Part print with two shaded views. Sizes in mm from the minimum x, y, z corner. Round coordinates to 2 decimals unless told otherwise and drop trailing zeros. Order: outer loops, then holes, each group sorted by start corner. A loop starts at its lowest first (then second) coordinate and runs counter-clockwise, first axis right, second up. Notation, with made-up numbers: (63, 26.25) - (85, 26.25) arc R28 ccw to (85, 62.25) - close; hole circle Ø4 at (85, 48.25). An arc over 180 degrees is marked (long way). Write item = value, one per line.
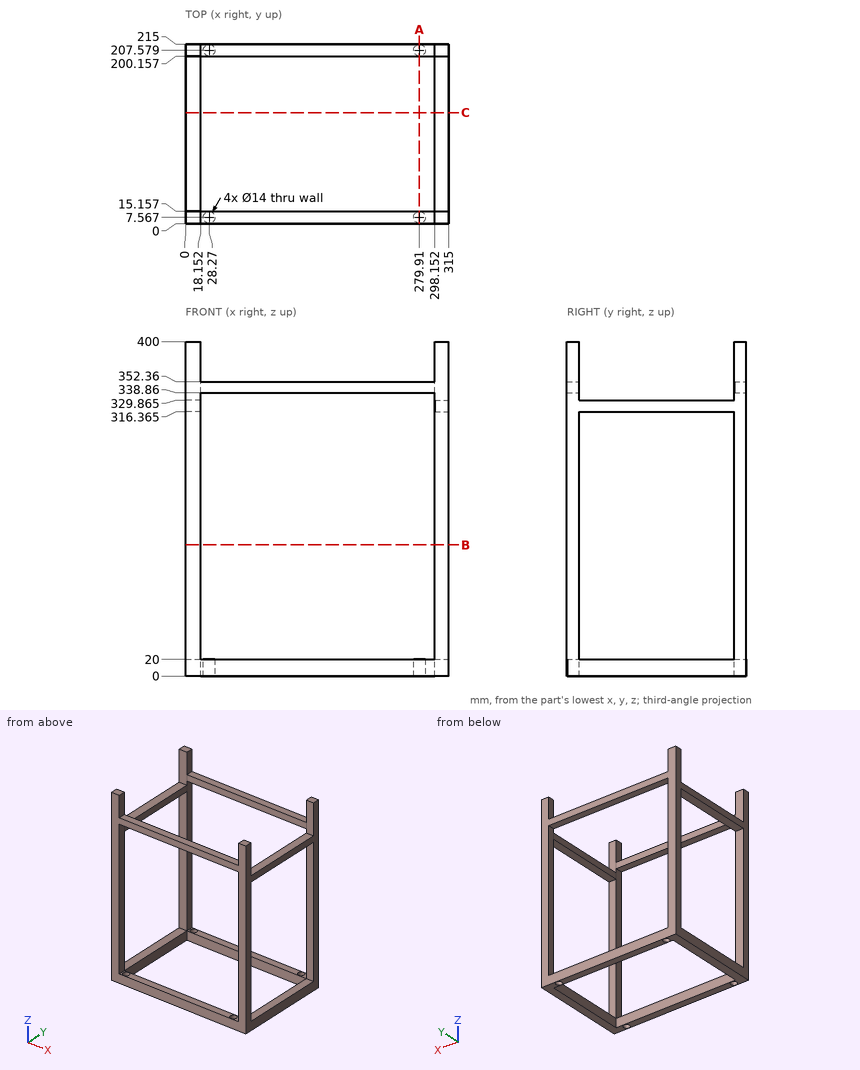
1) Flat gauge pin, fed straight in: pin 1 Ø13.5 at (x, y) = (310.5, 108) entering from +Z (3 decimals). Where does the tip first touch, or does it go through?
Conclusion:
pin_1 = 329.865
2) Cut at A-A (x = 279.91). Write the cut outline in (y, z).
Conclusion:
outline = (0, 0) - (0.57, 0) - (0.57, 20) - (0, 20) - close; (0, 338.86) - (15.16, 338.86) - (15.16, 352.36) - (0, 352.36) - close; (14.57, 0) - (15.16, 0) - (15.16, 20) - (14.57, 20) - close; (200.16, 0) - (200.58, 0) - (200.58, 20) - (200.16, 20) - close; (200.16, 338.86) - (215, 338.86) - (215, 352.36) - (200.16, 352.36) - close; (214.58, 0) - (215, 0) - (215, 20) - (214.58, 20) - close
3) Cut at C-C (y = 133). Write the cut outline in (x, z) (1 decimal).
Conclusion:
outline = (0, 0) - (18.2, 0) - (18.2, 20) - (0, 20) - close; (0, 316.4) - (18.2, 316.4) - (18.2, 329.9) - (0, 329.9) - close; (298.2, 0) - (315, 0) - (315, 20) - (298.2, 20) - close; (298.2, 316.4) - (315, 316.4) - (315, 329.9) - (298.2, 329.9) - close
4) Wall check: line 1 along Y through (x, z) = (28.27, 15.5); line 2 along Y through (x, z) = (279, 12); line 3 along Z through (x, y) = (100, 206.5). Give the ranges that are in metal, low to high.
Conclusion:
line_1 = 0 to 0.57, 14.57 to 15.16, 200.16 to 200.58, 214.58 to 215
line_2 = 0 to 0.63, 14.51 to 15.16, 200.16 to 200.64, 214.52 to 215
line_3 = 0 to 20, 338.86 to 352.36
5) Cut at B-B (z = 157). Write the cut outline in (x, y).
Conclusion:
outline = (0, 0) - (18.15, 0) - (18.15, 15.16) - (0, 15.16) - close; (0, 200.16) - (18.15, 200.16) - (18.15, 215) - (0, 215) - close; (298.15, 0) - (315, 0) - (315, 15.16) - (298.15, 15.16) - close; (298.15, 200.16) - (315, 200.16) - (315, 215) - (298.15, 215) - close
